Part model, mm, in its own coordinate system. A direction names the side the tool comes from. Give positions to 0.01 mm unless a question says otherwise; leave off trailing zeros. Write each loop counter-clockwise with the first axis right and the second up, starting at its lowest first coordinate (ties: lowest second). Pieces come first, ordered by that corner, then holes. Notation, with made-up numbers: (54, 60) - (109, 60) arc R23 cw to (109, 74) - close; hole circle Ø6 at (-24, 2). An arc over 180 degrees is marked (long way). Answer as a JSON object with one key per item and string values. Group by question number.
```python
from build123d import *

# Parameters (mm, degrees)
EXTRUDE_1_DEPTH = 24
SKETCH_2_R      = 1.15
EXTRUDE_2_DEPTH = 7
SKETCH_3_R      = 1.15
EXTRUDE_3_DEPTH = 4
SKETCH_4_R      = 3.1
EXTRUDE_4_DEPTH = 11
CHAMFER_4_SIZE  = 0.5
EXTRUDE_5_DEPTH = 0.5


with BuildPart() as part:
    # 草图1 → 凸台-拉伸1 (new body)
    with BuildSketch(Plane(origin=(0, 0, 0), x_dir=(0, 0, -1), z_dir=(1, 0, 0))):
        with BuildLine():
            Line((9.477737072, -8.15), (-9.477737072, -8.15))
            ThreePointArc((-9.477737072, -8.15), (-12.5, 0), (-9.477737072, 8.15))
            Line((-9.477737072, 8.15), (9.477737072, 8.15))
            ThreePointArc((9.477737072, 8.15), (12.5, 0), (9.477737072, -8.15))
        make_face()
    extrude(amount=EXTRUDE_1_DEPTH)

    # 草图2 → 凸台-拉伸2 (add)
    with BuildSketch(Plane.ZY):
        with BuildLine():
            Line((0, 4), (15.75, 4))
            ThreePointArc((15.75, 4), (19.75, 0), (15.75, -4))
            Line((15.75, -4), (0, -4))
            ThreePointArc((0, -4), (-4, 0), (0, 4))
        make_face()
        with Locations((15.75, 0)):
            Circle(SKETCH_2_R, mode=Mode.SUBTRACT)
    extrude(amount=-EXTRUDE_2_DEPTH)

    # 草图3 → 凸台-拉伸3 (add, symmetric)
    with BuildSketch(Plane(origin=(0, 0, 0), x_dir=(1, 0, 0), z_dir=(0, 1, 0))):
        with BuildLine():
            Line((0, 0), (0, 15.75))
            ThreePointArc((0, 15.75), (3.5, 19.25), (7, 15.75))
            Line((7, 15.75), (7, 0))
            ThreePointArc((7, 0), (3.5, -3.5), (0, 0))
        make_face()
        with Locations((3.5, 15.75)):
            Circle(SKETCH_3_R, mode=Mode.SUBTRACT)
    extrude(amount=EXTRUDE_3_DEPTH, both=True)

    # 草图4 → 凸台-拉伸4 (add)
    with BuildSketch(Plane.ZY):
        Circle(SKETCH_4_R)
    extrude(amount=EXTRUDE_4_DEPTH)

    # 倒角4
    chamfer_4_edges = [part.edges().sort_by_distance(p)[0] for p in [
        (24, 0, -12.5),
        (24, 8.15, 0),
        (24, 0, 12.5),
        (24, -8.15, 0),
    ]]
    chamfer(chamfer_4_edges, length=CHAMFER_4_SIZE)

    # 草图5 → 凸台-拉伸5 (add)
    with BuildSketch(Plane(origin=(24, 0, 0), x_dir=(0, 0, -1), z_dir=(1, 0, 0))):
        with BuildLine():
            Line((-9.556125253, 7.258131313), (8.461090538, -7.65))
            Line((8.461090538, -7.65), (-9.245404264, -7.65))
            ThreePointArc((-9.245404264, -7.65), (-11.997394419, -0.250054295), (-9.556125253, 7.258131313))
        make_face()
        with BuildLine():
            Line((9.245404264, 7.65), (-8.461090538, 7.65))
            Line((-8.461090538, 7.65), (9.556125253, -7.258131313))
            ThreePointArc((9.556125253, -7.258131313), (11.997394419, 0.250054295), (9.245404264, 7.65))
        make_face()
    extrude(amount=EXTRUDE_5_DEPTH)


solid = part.part
```
1) Band-saw the part on C-C (x = 21). List the corners of the cut face in (y, z), plus the area to 3 significant figures.
2) Which spindle directions (+Z, -Z, +X, -X, +Y, -Y) get a long thin tool onto all of the face, cutting with end or side? Do faces 1 (the flat face through (4, 4, -14)), 2 (the flat face through (12, 8.15, 0)), 3 (the flat face through (24, 1, 1)), 4 (the flat face through (24.5, -2, 4)), 5 (the flat face through (3, -4, 14)). Say none if no direction does.
3) Band-saw the part on A-A (x = 3.5). List the corners of the cut face in (y, z), plus the area to 3 significant figures.
4) Mould opens along Z. For faces 6 (the cylindrical face through (3.42, 0.06, -19.25)), 7 (the conical face through (23.865, -0.121, 12.135)), 8 (the flat face through (12, -8.15, 0)), 9 (the cylindrical face through (3.45, 0.05, 14.6)) say: pulls with the +Z half, pulls with the -Z half, needs draft (parallel to the pull), parting line crosses it, or undercut.
5) Drop flat-ended pins along their axis: P1, Ø2, axis at x = 3.5, z = 13.5, coming from the -Y side; P2, Ø4, axis at x = 4.5, z = -14.5, coming from the +Y side; P3, Ø1.2, axis at y = 1, z = -14.5, coming from the +X side. Give the stop position or say it passes through.
6) Band-saw the part on D-D (z = 13). List the corners of the cut face in (x, y), plus the area to 3 significant figures.
7) Probe line 1 (Y direction, x = 1.75, z = 15.75); line 2 (X direction, y = -1.5, z = -15.75); line 3 (Z direction, x = 3.5, y = 1). List the from-to ranges inside material, lowest first.
8) Band-saw the part on B-B (z = 0). List the corners of the cut face in (x, y), plus the area to 3 significant figures.
Verdict:
{
 "1": {"outline": "(-8.15, -9.48) arc R12.5 ccw to (8.15, -9.48) - (8.15, 9.48) arc R12.5 ccw to (-8.15, 9.48) - close", "area": "376 mm2"},
 "2": {"face 1": "-Z, +X, -X, +Y", "face 2": "+Z, -Z, +X, -X, +Y", "face 3": "+X", "face 4": "+Z, -Z, +X, +Y, -Y", "face 5": "+Z, +X, -X, -Y"},
 "3": {"outline": "(-8.15, -9.48) arc R12.5 ccw to (-4, -11.84) - (-4, -14.6) - (4, -14.6) - (4, -11.84) arc R12.5 ccw to (8.15, -9.48) - (8.15, 9.48) arc R12.5 ccw to (4, 11.84) - (4, 15.75) arc R4 ccw to (-4, 15.75) - (-4, 11.84) arc R12.5 ccw to (-8.15, 9.48) - close; (-4, -19.25) - (4, -19.25) - (4, -16.9) - (-4, -16.9) - close; hole circle Ø2.3 at (0, 15.75)", "area": "462 mm2"},
 "4": {"face 6": "pulls with the -Z half", "face 7": "pulls with the +Z half", "face 8": "needs draft", "face 9": "undercut"},
 "5": {"P1": "y = -4", "P2": "y = 4", "P3": "x = 7"},
 "6": {"outline": "(0, -4) - (7, -4) - (7, 4) - (0, 4) - close", "area": "56.0 mm2"},
 "7": {"line 1": "-4 to -1.15, 1.15 to 4", "line 2": "0 to 2.35, 4.65 to 7", "line 3": "-19.25 to -16.9, -14.6 to 15.18, 16.32 to 19.62"},
 "8": {"outline": "(-11, -3.1) - (0, -3.1) - (0, -8.15) - (23.5, -8.15) - (24, -7.65) - (24.5, -7.65) - (24.5, -0.65) - (24, -0.65) - (24, 0.65) - (24.5, 0.65) - (24.5, 7.65) - (24, 7.65) - (23.5, 8.15) - (0, 8.15) - (0, 3.1) - (-11, 3.1) - close", "area": "466 mm2"}
}
